from build123d import *

# Parameters (mm, degrees)
SKETCH010_W   = 160
SKETCH010_H   = 160
PAD009_DEPTH  = 10
SKETCH011_R   = 34.1
SKETCH011_R_2 = 31.475436
PAD010_DEPTH  = 100


with BuildPart() as body011:
    # Sketch010 (on Face1 of CopyBoolean001) → Pad009 (new body)
    with BuildSketch(Plane.XY):
        with Locations((0.584024, 4.328783)):
            Rectangle(SKETCH010_W, SKETCH010_H)
    extrude(amount=PAD009_DEPTH)


with BuildPart() as motoradapter:
    # Sketch011 (on Face1 of CopyPad009) → Pad010 (new body)
    with BuildSketch(Plane.XY.offset(10)):
        Circle(SKETCH011_R)
        Circle(SKETCH011_R_2, mode=Mode.SUBTRACT)
    extrude(amount=PAD010_DEPTH)

    # Boolean002: union Body011
    add(body011.part)


solid = motoradapter.part
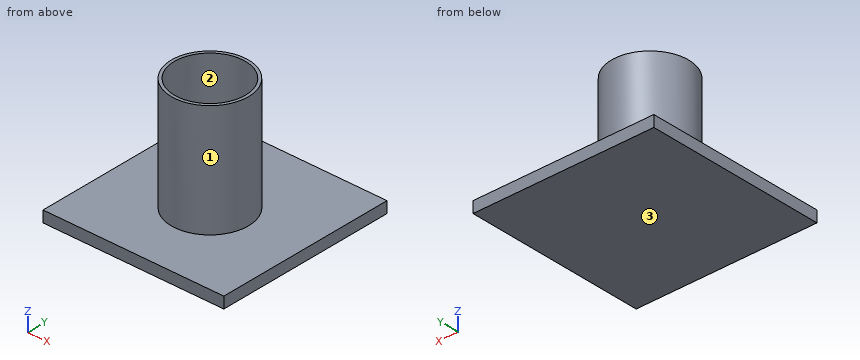
Source: CAD feature listing. Evaluate the final solid. Frame: model axes, mm. Face numbers are marked on the shaded views. Coordinates: 2 decimals unless noted, no trailing zeros. Loops run counter-clockwise (first coordinate to the right, second up) from the corner with the lowest first, then second, coordinate; pieces in that order, holes last. Notation, with made-up numbers: (-15, 26) -> (30, 26) arc R12 cw to (30, 46) -> close; hole circle Ø11 at (-10.75, -9.5). An arc over 180 degrees is marked (long way). Answer in a Markdown table with one row per item. Add a question column.
Q1. Ray query, line 1 along Y through (x, z) = (0, 39.5); line 2 along Z through (x, y) = (44.5, 22.5); line 3 along Y through (x, z) = (-7, 63). Return the intervals inside material, ascending.
Q2. Contact query for flat-ended pins moving along their axis: pin 1 Ø6 at (x, y) = (18, 34) entering from +Z; pin 2 Ø1 at (y, z) = (-31, 89.5) entering from +X; pin 3 Ø5 at (x, z) = (-11.5, 67) entering from +Y. Output: stop coordinate, or through.
Q3. Section D-D on x = 51. Return the cut outline in (y, z).
Q4. Pull-direction query (X, two-part tool) for the marked faces 1, 2 and 3; classes: pulls with the +X half, pulls with the -X half, needs draft (parallel to the pull), parting line crosses it, or undercut.
Q5. Section B-B on x = 0. Return the cut outline in (y, z).
Q6. Section C-C on z = 59. Return the cut outline in (x, y).
Q7. Section A-A on y = 0. Return the cut outline in (x, z).
Computed values:
| question | item | result |
|---|---|---|
| 1 | line 1 | y = -34.1 to -31.48, 31.48 to 34.1 |
| 1 | line 2 | z = 0 to 10 |
| 1 | line 3 | y = -33.37 to -30.69, 30.69 to 33.37 |
| 2 | pin 1 | stops at z = 10 |
| 2 | pin 2 | stops at x = 15.25 |
| 2 | pin 3 | stops at y = 32.89 |
| 3 | outline | (-75.67, 0) -> (84.33, 0) -> (84.33, 10) -> (-75.67, 10) -> close |
| 4 | face 1 | parting line crosses it |
| 4 | face 2 | undercut |
| 4 | face 3 | needs draft |
| 5 | outline | (-75.67, 0) -> (84.33, 0) -> (84.33, 10) -> (34.1, 10) -> (34.1, 110) -> (31.48, 110) -> (31.48, 10) -> (-31.48, 10) -> (-31.48, 110) -> (-34.1, 110) -> (-34.1, 10) -> (-75.67, 10) -> close |
| 6 | outline | circle Ø68.2 at (0, 0); hole circle Ø62.95 at (0, 0) |
| 7 | outline | (-79.42, 0) -> (80.58, 0) -> (80.58, 10) -> (34.1, 10) -> (34.1, 110) -> (31.48, 110) -> (31.48, 10) -> (-31.48, 10) -> (-31.48, 110) -> (-34.1, 110) -> (-34.1, 10) -> (-79.42, 10) -> close |
